from build123d import *

# Parameters (mm, degrees)
SKETCH1_R           = 7.5
SKETCH1_R_2         = 6
BOSS_EXTRUDE1_DEPTH = 9
FILLET1_R           = 0.3


with BuildPart() as part:
    # Sketch1 → Boss-Extrude1 (new body)
    with BuildSketch(Plane.XY):
        Circle(SKETCH1_R)
        Circle(SKETCH1_R_2, mode=Mode.SUBTRACT)
    extrude(amount=-BOSS_EXTRUDE1_DEPTH)

    # Fillet1
    fillet1_edges = [part.edges().sort_by_distance(p)[0] for p in [
        (-7.5, 0, 0),
        (-7.5, 0, -9),
        (-6, 0, -9),
        (-6, 0, 0),
    ]]
    fillet(fillet1_edges, radius=FILLET1_R)


solid = part.part
Geometry check sheet. Reference: the model listing, model coordinates, mm. Coordinates: 2 decimals unless noted, no trailing zeros. Order: outer loops, then holes, each group sorted by start corner. A loop starts at its lowest first (then second) coordinate and runs counter-clockwise, first axis right, second up. Notation, with made-up numbers: (-3, 1) - (19, 1) arc R21 ccw to (19, 29) - close; hole circle Ø5 at (58.25, -32.5). An arc over 180 degrees is marked (long way). Answer in a Markdown table with one row per item. Add a question column.
1) Material ranges on line 1 along Y through (x, z) = (0, -2); line 2 along Y through (x, z) = (4.5, -2.75); line 3 along X through (y, z) = (-4.75, -7), recorded low to high. Write a range as [from, to].
2) Gauge pin test, flat ends, axial feed: P1, Ø3, axis at x = -2.5, z = -3.5, coming from the -Y side; P2, Ø3, axis at x = 6, y = 0, coming from the +Z side; P3, Ø5, axis at y = -4, z = -1, coming from the -X side; P4, Ø2, axis at y = 5.5, z = -6.5, coming from the +X side. Record the tip position at first contact, or that the pin passes through.
3) Cross-section at A-A, the plane y = 0. Record the cut outline in (x, z), then the cut area to 3 significant figures.
4) Release check for a two-part mould opening along Y. For faces 1 (the flat face through (3, -6, -9)), 2 (the cylindrical face through (-7.493, 0.33, -4.441)), 3 (the cylindrical face through (-6, 0, -4)) record: +Y half, -Y half, draft (parallel to the pull), parting line (faces both ways), or undercut.
5) Cross-section at C-C, the plane z = -7. Record the cut outline in (x, y), then the cut area to 3 significant figures.
Check result:
| question | item | result |
|---|---|---|
| 1 | line 1 | y = [-7.5, -6], [6, 7.5] |
| 1 | line 2 | y = [-6, -3.97], [3.97, 6] |
| 1 | line 3 | x = [-5.8, -3.67], [3.67, 5.8] |
| 2 | P1 | stops at y = -7.43 |
| 2 | P2 | stops at z = 0 |
| 2 | P3 | stops at x = -7.35 |
| 2 | P4 | stops at x = 6 |
| 3 | outline | (-7.5, -8.7) arc R0.3 ccw to (-7.2, -9) - (-6.3, -9) arc R0.3 ccw to (-6, -8.7) - (-6, -0.3) arc R0.3 ccw to (-6.3, 0) - (-7.2, 0) arc R0.3 ccw to (-7.5, -0.3) - close; (6, -8.7) arc R0.3 ccw to (6.3, -9) - (7.2, -9) arc R0.3 ccw to (7.5, -8.7) - (7.5, -0.3) arc R0.3 ccw to (7.2, 0) - (6.3, 0) arc R0.3 ccw to (6, -0.3) - close |
| 3 | area | 26.8 mm² |
| 4 | face 1 | draft |
| 4 | face 2 | parting line |
| 4 | face 3 | undercut |
| 5 | outline | circle Ø15 at (0, 0); hole circle Ø12 at (0, 0) |
| 5 | area | 63.6 mm² |
